```python
from build123d import *

# Parameters (mm, degrees)
F1_DEPTH    = 2.5
F2_R        = 5
F3_T1_DEPTH = 5


# Not quite as in the source:
# - a fillet or chamfer that OpenCascade refuses, or shapes differently, is made with other operations: its cross-section is extruded or revolved along the edge and cut away or added


with BuildPart() as f1:
    # F0 (on Front) → F1 (new body, symmetric)
    with BuildSketch(Plane.XZ):
        with BuildLine():
            Line((18.5, 12), (-18.5, 12))
            Line((-18.5, 12), (-18.5, -12))
            Line((-18.5, -12), (18.5, -12))
            Line((18.5, -12), (18.5, -4))
            Line((18.5, -4), (15.5, -4))
            Line((15.5, -4), (15.5, -9))
            Line((15.5, -9), (-12.5, -9))
            Line((-12.5, -9), (-12.5, -1.5))
            ThreePointArc((-12.5, -1.5), (-15.714868952, 0), (-12.5, 1.5))
            Line((-12.5, 1.5), (-12.5, 9))
            Line((-12.5, 9), (15.5, 9))
            Line((15.5, 9), (15.5, 4))
            Line((15.5, 4), (18.5, 4))
            Line((18.5, 4), (18.5, 12))
        make_face()
    extrude(amount=F1_DEPTH, both=True)

    # F2
    f2_edges = [f1.edges().sort_by_distance(p)[0] for p in [
        (-18.5, 0, 12),
        (18.5, 0, 12),
        (18.5, 0, -12),
        (-18.5, 0, -12),
    ]]
    fillet(f2_edges, radius=F2_R)

    # F3: fillet of radius 7 on 4 edges, made by hand

    # F3_s2 → F3_t1 (join)
    with BuildSketch(Plane.XZ.offset(-2.5)):
        with BuildLine():
            ThreePointArc((15.5, 4), (12.9750962002, 7.6124860802), (8.7917960675, 9))
            Line((8.7917960675, 9), (15.5, 9))
            Line((15.5, 9), (15.5, 4))
        make_face()
        with BuildLine():
            ThreePointArc((15.5, -4), (12.9750962002, -7.6124860802), (8.7917960675, -9))
            Line((8.7917960675, -9), (15.5, -9))
            Line((15.5, -9), (15.5, -4))
        make_face()
        with BuildLine():
            ThreePointArc((-12.5, -2), (-10.4497474683, -6.9497474683), (-5.5, -9))
            Line((-5.5, -9), (-12.5, -9))
            Line((-12.5, -9), (-12.5, -2))
        make_face()
        with BuildLine():
            ThreePointArc((-5.5, 9), (-10.4497474683, 6.9497474683), (-12.5, 2))
            Line((-12.5, 2), (-12.5, 9))
            Line((-12.5, 9), (-5.5, 9))
        make_face()
    extrude(amount=F3_T1_DEPTH)


solid = f1.part
```
Check sheet for the modelled part. Datum: model origin and axes. Units: mm. A direction names the side the tool comes from. Give positions to 0.01 mm unless a question says otherwise; leave off trailing zeros. Write each loop counter-clockwise with the first axis right and the second up, starting at its lowest first coordinate (ties: lowest second). Pieces come first, ordered by that corner, then holes.
Item 1: Cross-section at D-D (z = 0). Enter the section's corners in (x, y).
Item 2: Access from +Z, -Z, +X, -X, +Y, -Y to the whole of each face (thin tool, end or side, straight path). Record for faces 1 (the face through (17, 0, -4)), 2 (the face through (-17, -0.04, -10.57)), 3 (the face through (2, 0, 9)).
Item 3: Cross-section at A-A (x = -3). Enter the section's corners in (y, z), and give its area (3 significant figures).
Item 4: Scan lines: L1, parallel to Z at x = 0.5, y = -2; L2, parallel to Z at x = 16.5, y = 1.65; L3, parallel to X at y = 1.5, z = -5.5. Record each from-to range of solid material in increasing order.
Item 5: Cross-section at B-B (z = -6.25). Enter the section's corners in (x, y), and give its area (3 significant figures).
Item 6: Draft check along Z on faces 4 (the face through (0, 0, 12)), 5 (the face through (-15.714, -0.035, -0.062)), 6 (the face through (18.5, 0, 5)). Enter one of: released by +Z, released by -Z, zero draft, split by the parting line, or undercut.
Item 7: Cross-section at C-C (y = 1.75). Enter the section's corners in (x, z), and give its area (3 significant figures).
Item 8: Gauge pin test, flat ends, axial feed: pin 1 (0.6 mm diameter, centred on y = 0.5, z = -2, fed in from +X); pin 2 (1.5 mm diameter, centred on y = 0.5, z = -8.5, fed in from +X); pin 3 (0.9 mm diameter, centred on x = 16.5, y = -1, fed in from +Z). Record the tip position at first contact, or that the pin passes through.
Report:
1. outline: (-18.5, -2.5) - (-15.71, -2.5) - (-15.71, 2.5) - (-18.5, 2.5) - close
2. face 1: +X, +Y, -Y
2. face 2: -Z, -X, +Y, -Y
2. face 3: +Y, -Y
3. outline: (-2.5, -12) - (2.5, -12) - (2.5, -9) - (-2.5, -9) - close; (-2.5, 9) - (2.5, 9) - (2.5, 12) - (-2.5, 12) - close
3. area: 30.0 mm2
4. L1: z = -12 to -9, 9 to 12
4. L2: z = -11 to -4, 4 to 11
4. L3: x = -18.5 to -11.56, 14.85 to 18.5
5. outline: (-18.5, -2.5) - (-11.06, -2.5) - (-11.06, 2.5) - (-18.5, 2.5) - close; (14.35, -2.5) - (18.5, -2.5) - (18.5, 2.5) - (14.35, 2.5) - close
5. area: 57.9 mm2
6. face 4: released by +Z
6. face 5: undercut
6. face 6: zero draft
7. outline: (-18.5, -7) arc R5 ccw to (-13.5, -12) - (13.5, -12) arc R5 ccw to (18.5, -7) - (18.5, -4) - (15.5, -4) arc R7 cw to (8.79, -9) - (-5.5, -9) arc R7 cw to (-12.5, -2) - (-12.5, -1.5) arc R1.96 cw (long way) to (-12.5, 1.5) - (-12.5, 2) arc R7 cw to (-5.5, 9) - (8.79, 9) arc R7 cw to (15.5, 4) - (18.5, 4) - (18.5, 7) arc R5 ccw to (13.5, 12) - (-13.5, 12) arc R5 ccw to (-18.5, 7) - close
7. area: 367 mm2
8. pin 1: stops at x = -12.49
8. pin 2: stops at x = 18.44
8. pin 3: stops at z = 11.3
